Design review of the part built by this model. Coordinates are the model's own, in mm. A direction names the side the tool comes from. Round coordinates to 2 decimals unless told otherwise and drop trailing zeros. Loops run counter-clockwise (first coordinate to the right, second up) from the corner with the lowest first, then second, coordinate; pieces in that order, holes last. Notation, with made-up numbers: (82, 46) - (107, 46) arc R11 cw to (107, 50) - close; hole circle Ø6 at (23, -1). An arc over 180 degrees is marked (long way). Answer as CSV lines item,"result". Start each with the question number.
(1) Mouldability with a two-part tool opening along Z and no side actions: class faces 1 (the cylindrical face through (44.859, 70.328, -20.547)), 2 (the flat face through (-1, 29, 4)), 3 (the cylindrical face through (14.93, 70.27, -15.25)) as released by +Z, released by -Z, zero draft, split by the parting line, or undercut.
(2) For faces 4 (the flat face through (-1, 25, 4)), 5 (the flat face through (11.75, 70, -7)), 6 (the cylindrical face through (-0.644, 71.097, 10.609)), 7 (the flat face through (-1, 13, -4)), 8 (the flat face through (-1, 48, 7.75)), list the 3-axis set-ups (+Z, -Z, +X, -X, +Y, -Y) from which the entire face can be reached by the end or side of a thin tool; tool diameter is ignored.
(3) Consider section B-B (y = 18). Give the boundary of the cut face in (x, z).
(4) For P1, Ø12, axis at x = -32, z = 8, coming from the -Y side; P2, Ø10, axis at x = -10.5, y = 48.5, coming from the -Z side; P3, Ø7.5, axis at x = -1, y = 17, coming from the -Z side; P4, Ø3.5, axis at x = 40, y = 18, coming from the -Z side, all flat-tipped, find the tip position at first contact; note any pin that passes through.
(5) Consider section C-C (z = -5.5). Give the boundary of the cut face in (x, y).
(6) Consider section D-D (x = -21). Give the boundary of the cut face in (y, z), and give its area (3 significant figures).
(7) Wall thickness on L1, parallel to Y at x = -40, z = -1.7; L2, parallel to Y at x = 23, z = 2.5; L3, parallel to Y at x = -40, z = -2.05: over which ranges is each line inside the solid? List them lowest first.
(8) Consider section A-A (x = 40). Give the boundary of the cut face in (y, z).
Autodesk Fusion 360 part; units mm, degrees
sketch "Sketch5" plane through (0, 0, 0) normal (0, 0, 1) x (1, 0, 0)
  line L0 (-40, 6) -> (40, 6) construction
  line L1 (40, 6) -> (40, 18) construction
  line L2 (40, 18) -> (-40, 18) construction
  line L3 (-40, 18) -> (-40, 6) construction
  circle A0 centre (-40, 18) radius 2.25
  circle A1 centre (-40, 6) radius 2.25
  circle A2 centre (40, 18) radius 2.25
  circle A3 centre (40, 6) radius 2.25
  line L4 (46, 24) -> (-46, 24)
  line L5 (-46, 24) -> (-46, 0)
  line L6 (-46, 0) -> (46, 0)
  line L7 (46, 0) -> (46, 24)
  line L8 (46, 24) -> (46, 25)
  line L9 (46, 25) -> (-46, 25)
  line L10 (-46, 25) -> (-46, 24)
  dimension "d20" = 80
  dimension "d21" = 12
  dimension "d22" = 4.5
  dimension "d42" = 6
  dimension "d56" = 92
  dimension "d70" = 1
  dimension "d71" = 25
extrude "Extrude6" add sketch "Sketch5" against normal blind 4
sketch "Sketch9" plane through (0, 0, 0) normal (1, 0, 0) x (0, 1, 0)
  line L0 (25, -4) -> (29, -4)
  line L1 (29, -4) -> (29, 7.75)
  line L2 (29, 7.75) -> (68.3, 7.75)
  line L3 (68.3, 7.75) -> (68.3, -21.75)
  line L4 (68.3, -21.75) -> (72.3, -21.75)
  line L5 (72.3, -21.75) -> (72.3, 11.75)
  line L6 (72.3, 11.75) -> (25, 11.75)
  line L7 (25, 11.75) -> (25, 0)
  line L8 (25, 0) -> (29, 0) construction
  line L9 (48.65, 7.75) -> (48.65, 11.75) construction
  line L10 (25, 0) -> (25, -4)
  line L11 (25, -4) -> (25, 0)
  line L12 (0, 0) -> (25, 0)
  line L13 (25, 0) -> (25, -4)
  line L14 (25, -4) -> (0, -4)
  line L15 (0, -4) -> (0, 0)
  point P0 (68.3, -7)
  dimension "d52" = 7
  dimension "d53" = 14.75
  dimension "d55" = 14.75
  dimension "d72" = 72.3
extrude "Extrude7" add sketch "Sketch9" along normal mid plane 92 contours L0 L1 L2 L3 L4 L5 L6 L7 L10 L11 L13
fillet "Fillet3" radius 4 7 edges at (46, 70.3, -21.75) (-46, 70.3, -21.75) (0, 72.3, 11.75) (0, 25, 11.75) (0, 29, -4) (-46, 0, -2) (46, 0, -2)
sketch "Sketch10" plane through (0, 0, 0) normal (0, 1, 0) x (1, 0, 0)
  line L0 (15, 2) -> (15, 12) construction
  arc A0 (18.25, 11.9963) -> (11.75, 12) centre (15, 12) ccw
  arc A1 (11.75, 2.0001) -> (18.25, 2) centre (15, 2) ccw
  line L1 (11.75, 12) -> (11.75, 2.0001)
  line L2 (18.25, 2) -> (18.25, 11.9963)
  line L3 (15, 7) -> (0, 7) construction
  point P0 (0, 7)
  dimension "d63" = 10
  dimension "d64" = 3.25
  dimension "d68" = 15
extrude "Extrude8" cut sketch "Sketch10" along normal through all from surface at 68.3
equation "Thickness = 4 mm"
equation "d52 = ( MountHoleSpacing - 148 mm ) / 2"
equation "d53 = ( ( MountHoleTolerance + MountHoleSize ) / 2 ) + MountHoleSize"
equation "d55 = d53"
equation "d57 = d56"
equation "d60 = Thickness"
equation "MountHoleSpacing = 162 mm"
equation "MountHoleTolerance = 10 mm"
equation "d63 = MountHoleTolerance"
equation "d64 = ( 6.5 / 2 ) * 1 mm"
equation "MountHoleSize = 6.5 mm"
equation "SurfaceOffset = 30 mm"
equation "d72 = 42.3 mm + SurfaceOffset"
Determined:
1,face 1,"released by -Z"
1,face 2,"zero draft"
1,face 3,"undercut"
2,face 4,"+Z, +X, -X, -Y"
2,face 5,"+Y"
2,face 6,"+Z, +X, -X, +Y"
2,face 7,"-Z, +X, -X, -Y"
2,face 8,"-Z, +X, -X"
3,outline,"(-46, -4) - (-42.25, -4) - (-42.25, 0) - (-46, 0) - close; (-37.75, -4) - (37.75, -4) - (37.75, 0) - (-37.75, 0) - close; (42.25, -4) - (46, -4) - (46, 0) - (42.25, 0) - close"
4,P1,"stops at y = 25"
4,P2,"stops at z = 7.75"
4,P3,"stops at z = -4"
4,P4,"passes through"
5,outline,"(-46, 68.3) - (11.75, 68.3) - (11.75, 72.3) - (-46, 72.3) - close; (18.25, 68.3) - (46, 68.3) - (46, 72.3) - (18.25, 72.3) - close"
6,outline,"(0, -4) - (25, -4) arc R4 ccw to (29, 0) - (29, 7.75) - (68.3, 7.75) - (68.3, -21.75) - (72.3, -21.75) - (72.3, 7.75) arc R4 ccw to (68.3, 11.75) - (29, 11.75) arc R4 ccw to (25, 7.75) - (25, 0) - (0, 0) - close"
6,area,"444 mm^2"
7,L1,"y = 0 to 3.75, 8.25 to 15.75, 20.25 to 28.62, 68.3 to 72.3"
7,L2,"y = 25 to 29, 68.3 to 72.3"
7,L3,"y = 0 to 3.75, 8.25 to 15.75, 20.25 to 28.43, 68.3 to 72.3"
8,outline,"(0, -4) - (3.75, -4) - (3.75, 0) - (0, 0) - close; (8.25, -4) - (15.75, -4) - (15.75, 0) - (8.25, 0) - close; (20.25, -4) - (25, -4) arc R4 ccw to (29, 0) - (29, 7.75) - (68.3, 7.75) - (68.3, -21.75) - (72.3, -21.75) - (72.3, 7.75) arc R4 ccw to (68.3, 11.75) - (29, 11.75) arc R4 ccw to (25, 7.75) - (25, 0) - (20.25, 0) - close"
